Study the drawing (mm; zero at the part's minimum x, y, z) and answer. Round coordinates to 2 decimals unless told otherwise and drop trailing zeros. Order: outer loops, then holes, each group sorted by start corner. A loop starts at its lowest first (then second) coordinate and runs counter-clockwise, first axis right, second up. Notation, with made-up numbers: M 85,-9.75 L 144,-9.75 A23 cw 144,2.25 Z; hole C 21,-25.75 d6. An arc over 180 degrees is marked long. Put each result on its own line as item: value. Start each with the question number.
1. Each of these flat-tipped pins is pushed along its axis until it touches: pin 1 Ø1 at (y, z) = (86.5, 3) entering from +X; pin 2 Ø10 at (x, y) = (21.5, 27) entering from -Z. Where does it stop, or does it pass through?
2. The part is cut by section D-D (x = 167). Give the vertices of the cut face in (y, z) (1 decimal), then the cut area to 3 significant figures.
3. The part is cut by section C-C (y = 14). Give the vertices of the cut face in (x, z) (1 decimal).
4. Consider line 1 (Y direction, x = 93.98, z = 1.55); line 2 (Y direction, x = 106, z = 0.4); line 3 (X direction, y = 118, z = 0.95). Determine where each line is inside the solid, lowest interval first.
5. The part is cut by section A-A (y = 93.98). Give the vertices of the cut face in (x, z) (3 decimals).
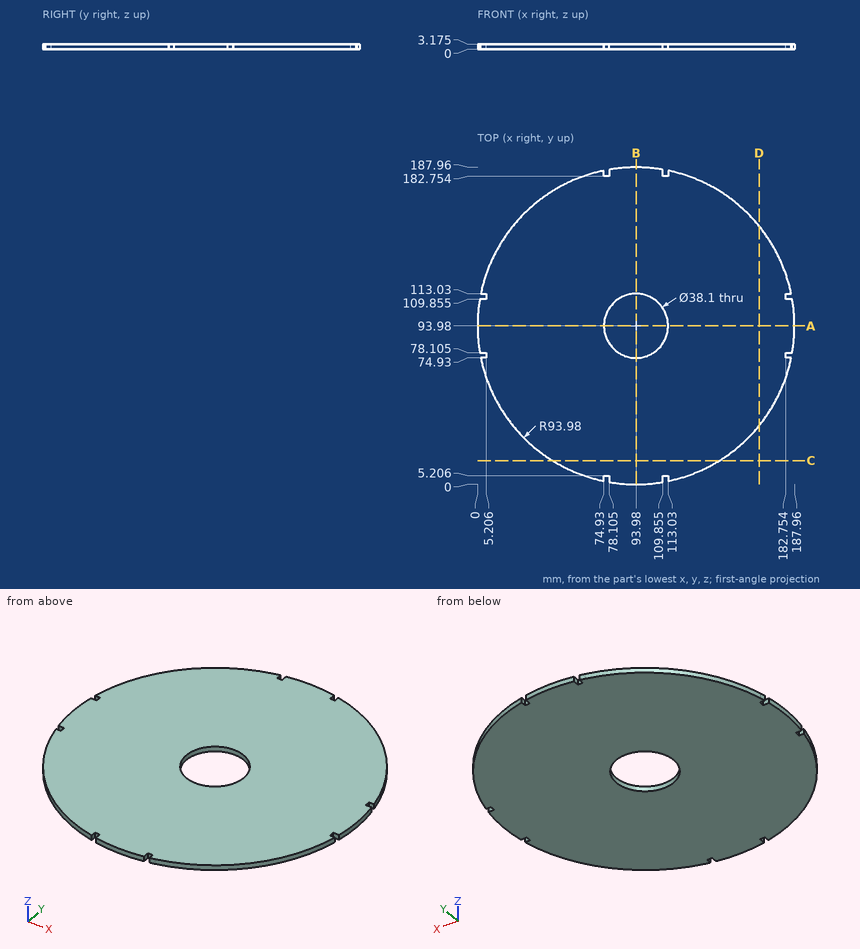
Resolved:
1. pin 1: x = 187.7
1. pin 2: z = 0
2. outline: M 34.8,0 L 153.1,0 L 153.1,3.2 L 34.8,3.2 Z
2. area: 376 mm2
3. outline: M 44.6,0 L 143.3,0 L 143.3,3.2 L 44.6,3.2 Z
4. line 1: 0 to 74.93, 113.03 to 187.96
4. line 2: 0.77 to 79.2, 108.76 to 187.19
4. line 3: 3.12 to 184.84
5. outline: M 0,0 L 74.93,0 L 74.93,3.175 L 0,3.175 Z; M 113.03,0 L 187.96,0 L 187.96,3.175 L 113.03,3.175 Z
